Autodesk Inventor part; units mm, degrees
ref_plane "YZ Plane" through (0, 0, 0) normal (1, 0, 0) x (0, 1, 0)
ref_plane "XZ Plane" through (0, 0, 0) normal (0, 1, 0) x (-1, 0, 0)
ref_plane "XY Plane" through (0, 0, 0) normal (0, 0, 1) x (1, 0, 0)
sketch "Sketch1" plane through (0, 0, 0) normal (0, 0, 1) x (1, 0, 0)
  arc A0 (18.6268, 80) -> (52, 10) centre (115.8042, 83.3748) ccw
  line L0 (0, 80) -> (18.6268, 80)
  line L1 (46.5, 0) -> (27.071, 0)
  line L2 (7.071, 0) -> (0, 0)
  line L3 (7.071, 0) -> (7.071, -45)
  line L4 (7.071, -45) -> (27.071, -45)
  line L5 (27.071, -45) -> (27.071, 0)
  line L6 (46.5, 0) -> (46.5, -60)
  line L7 (46.5, -60) -> (52, -60)
  line L8 (52, -60) -> (52, 0)
  line L9 (0, 80) -> (0, 0)
  line L10 (52, 10) -> (52, 0)
  dimension "d22" = 52
  dimension "d23" = 19.429
  dimension "d24" = 45
  dimension "d25" = 60
extrude "Extrusion2" add sketch "Sketch1" along normal blind 5.5
properties part number "brazos"
Geometry: final body of the model. Coordinates: model frame, mm. A direction names the side the tool comes from. Give positions to 0.01 mm unless a question says otherwise; leave off trailing zeros. Write each loop counter-clockwise with the first axis right and the second up, starting at its lowest first coordinate (ties: lowest second). Pieces come first, ordered by that corner, then holes. Notation, with made-up numbers: M 62.25,-8 L 102.25,-8 A6 cw 102.25,1 Z; hole C 29,-40 d5. An arc over 180 degrees is marked long. Answer in a Markdown table with one row per item. Add a question column.
(1) First-contact query: pin 1 (1.6 mm diameter, centred on y = -19, z = 4, fed in from -X); pin 2 (6 mm diameter, centred on x = 25.5, y = 58.5, fed in from -Z); pin 3 (2 mm diameter, centred on x = 41, z = 3, fed in from +Y); pin 4 (3 mm diameter, centred on x = 19.5, z = 3.5, fed in from -Y). Flat tips, straight axial feed; report the tip coordinate or a pass-through.
(2) Section B-B on z = 1.75. Return loops of the section in (x, y).
(3) Ray query, line 1 (X direction, y = -5, z = 1.5); line 2 (Y direction, x = 7.5, z = 2.95); line 3 (Y direction, x = 5, z = 1.85). Return the intervals inside material, ascending.
(4) Section C-C on x = 14. Return loops of the section in (y, z).
(5) Mould query, pull axis X, two halves, no side actions, for faces 4 (the flat face through (9, 80, 3)), 5 (the flat face through (46.5, -30, 3)), 6 (the flat face through (7.071, -22, 3)), 7 (the flat face through (37, 0, 3)). Classes: +X half, -X half, draft (parallel to the pull), parting line (faces both ways), or undercut.
(6) Section D-D on y = 55.5. Return loops of the section in (x, z).
(7) Section A-A on y = -9. Return loops of the section in (x, z), and give its area (3 significant figures).
(8) Reachability of faces 1 (the flat face through (17, -45, 3)), 2 (the flat face through (27.071, -23, 3)), 3 (the cylindrical face through (28.275, 41.026, 2.712)) from +Z, -Z, +X, -X, +Y, -Y: full face, straight path, thin tool, end or side. Return the list, or none.
Result set:
| question | item | result |
|---|---|---|
| 1 | pin 1 | stops at x = 7.07 |
| 1 | pin 2 | passes through |
| 1 | pin 3 | stops at y = 22.48 |
| 1 | pin 4 | stops at y = -45 |
| 2 | outline | M 0,0 L 7.07,0 L 7.07,-45 L 27.07,-45 L 27.07,0 L 46.5,0 L 46.5,-60 L 52,-60 L 52,10 A97.24 cw 18.63,80 L 0,80 Z |
| 3 | line 1 | x = 7.07 to 27.07, 46.5 to 52 |
| 3 | line 2 | y = -45 to 80 |
| 3 | line 3 | y = 0 to 80 |
| 4 | outline | M -45,0 L 80,0 L 80,5.5 L -45,5.5 Z |
| 5 | face 4 | draft |
| 5 | face 5 | undercut |
| 5 | face 6 | -X half |
| 5 | face 7 | undercut |
| 6 | outline | M 0,0 L 22.65,0 L 22.65,5.5 L 0,5.5 Z |
| 7 | outline | M 7.07,0 L 27.07,0 L 27.07,5.5 L 7.07,5.5 Z; M 46.5,0 L 52,0 L 52,5.5 L 46.5,5.5 Z |
| 7 | area | 140 mm^2 |
| 8 | face 1 | +Z, -Z, -X, -Y |
| 8 | face 2 | +Z, -Z, -Y |
| 8 | face 3 | +Z, -Z, +X, +Y |
